```python
from build123d import *

# Parameters (mm, degrees)
BOSS_EXTRUDE1_DEPTH = 30
SKETCH2_R           = 5
CUT_EXTRUDE1_DEPTH  = 90
FILLET1_R           = 15
SKETCH3_W           = 67
SKETCH3_H           = 30
BOSS_EXTRUDE2_DEPTH = 20
BOSS_EXTRUDE2_TAPER = 11
SKETCH4_R           = 5
CUT_EXTRUDE2_DEPTH  = 5


with BuildPart() as part:
    # Sketch1 → Boss-Extrude1 (new body)
    with BuildSketch(Plane.XY):
        Polygon((0, 0), (30.5, 0), (30.5, 37), (33.5, 37), (33.5, -3), (0, -3), align=None)
    boss_extrude1 = extrude(amount=BOSS_EXTRUDE1_DEPTH)

    # Mirror1: Boss-Extrude1 across plane
    add(boss_extrude1.mirror(Plane(origin=(0, -3, 30), x_dir=(0, 0, 1), z_dir=(1, 0, 0))))

    # Sketch2 → Cut-Extrude1 (cut)
    with BuildSketch(Plane.ZY.offset(33.5)):
        with Locations((15, 17)):
            Circle(SKETCH2_R)
    extrude(amount=-CUT_EXTRUDE1_DEPTH, mode=Mode.SUBTRACT)

    # Fillet1
    fillet1_edges = [part.edges().sort_by_distance(p)[0] for p in [
        (-32, 37, 30),
        (-32, 37, 0),
        (32, 37, 0),
        (32, 37, 30),
    ]]
    fillet(fillet1_edges, radius=FILLET1_R - 0.0001)  # a hair under: the kernel refuses the full size

    # Sketch3 → Boss-Extrude2 (add)
    with BuildSketch(Plane.XZ.offset(3)):
        with Locations((0, 15)):
            Rectangle(SKETCH3_W, SKETCH3_H)
    extrude(amount=BOSS_EXTRUDE2_DEPTH, taper=BOSS_EXTRUDE2_TAPER)

    # Sketch4 → Cut-Extrude2 (cut)
    with BuildSketch(Plane.XZ.offset(23)):
        with Locations((0, 15)):
            Circle(SKETCH4_R)
    extrude(amount=-CUT_EXTRUDE2_DEPTH, mode=Mode.SUBTRACT)


solid = part.part
```
The listing builds one solid part. Answer for the finished solid, in the listing's coordinates (mm). A direction names the side the tool comes from. Round coordinates to 2 decimals unless told otherwise and drop trailing zeros. Loops run counter-clockwise (first coordinate to the right, second up) from the corner with the lowest first, then second, coordinate; pieces in that order, holes last.
1) A cutting plane is placed at B-B on y = 1.5. Determine the outline of the cut face in (x, z), plus the area to 3 significant figures.
Outcome:
outline: (-33.5, 0) - (-30.5, 0) - (-30.5, 30) - (-33.5, 30) - close; (30.5, 0) - (33.5, 0) - (33.5, 30) - (30.5, 30) - close
area: 180 mm2
2) For faces 5 (the face through (0, -2, 30)), 6 (the face through (-30.5, 22.4, 14.8)), 7 (the face through (-1.08, -20.54, 10.12)), determine the directions among +Z, -Z, +X, -X, +Y, -Y from which every point of the face is accessible in a straight line to the end or side of a thin tool.
Outcome:
face 5: +Z, +X, -X, +Y, -Y
face 6: +Z, -Z, +Y
face 7: -Y
3) For a pull along Z with two mould halves and no side action, classify faces 1 (the face through (-32.02, 32.49, 4.28)), 2 (the face through (0, -18, 15)), 3 (the face through (-33.5, 12.8, 18.1)), 4 (the face through (-32.021, 12.564, 17.307)) as released by +Z, released by -Z, zero draft, split by the parting line, or undercut.
Outcome:
face 1: released by -Z
face 2: undercut
face 3: zero draft
face 4: undercut
4) A cutting plane is placed at C-C on y = 33. Determine the outline of the cut face in (x, z).
Outcome:
outline: (-33.5, 4.8) - (-30.5, 4.8) - (-30.5, 25.2) - (-33.5, 25.2) - close; (30.5, 4.8) - (33.5, 4.8) - (33.5, 25.2) - (30.5, 25.2) - close
5) Consider line 1 (X direction, y = 31, z = 13); line 2 (Y direction, x = -2, z = 4); line 3 (X direction, y = -7, z = 15.5). Determine where each line is inside the solid, lowest interval first.
Outcome:
line 1: x = -33.5 to -30.5, 30.5 to 33.5
line 2: y = -23 to 0
line 3: x = -32.72 to 32.72
6) A cutting plane is placed at D-D on z = 13. Give the number of separate pieces and of enclosed holes in the cut face, plus the area to 3 significant figures.
Outcome:
separate pieces: 3
enclosed holes: 0
area: 1,580 mm2
7) A cutting plane is placed at A-A on y = 17. Determine the outline of the cut face in (x, z), plus the area to 3 significant figures.
Outcome:
outline: (-33.5, 0) - (-30.5, 0) - (-30.5, 10) - (-33.5, 10) - close; (-33.5, 20) - (-30.5, 20) - (-30.5, 30) - (-33.5, 30) - close; (30.5, 0) - (33.5, 0) - (33.5, 10) - (30.5, 10) - close; (30.5, 20) - (33.5, 20) - (33.5, 30) - (30.5, 30) - close
area: 120 mm2
8) Given P1, Ø9, axis at x = 0, z = 15, coming from the +Y side; P2, Ø5, axis at x = -2, z = 15, coming from the -Y side, each flat-ended and moving along its own axis, determine where each tip first touches the part or whether it passes through.
Outcome:
P1: stops at y = 0
P2: stops at y = -18
